Here's how the part is built. I have some questions about the finished solid (model axes, mm). Coordinates: 2 decimals unless noted, no trailing zeros. Write each loop counter-clockwise with the first axis right and the second up, starting at its lowest first coordinate (ties: lowest second). Pieces come first, ordered by that corner, then holes.
```python
from build123d import *

# Parameters (mm, degrees)
SKETCH1_R           = 2.25
BOSS_EXTRUDE1_DEPTH = 3.18


with BuildPart() as part:
    # Sketch1 → Boss-Extrude1 (new body)
    with BuildSketch(Plane.XY):
        with BuildLine():
            ThreePointArc((22.5, 0), (15.998046756, 15.821267332), (0.25, 22.498611068))
            Line((0.25, 22.498611068), (0.25, -22.498611068))
            ThreePointArc((0.25, -22.498611068), (15.998046756, -15.821267332), (22.5, 0))
        make_face()
        with Locations(Location((9.25, -16.02146997, 0), (0, 0, 180))):
            Circle(SKETCH1_R, mode=Mode.SUBTRACT)
        with Locations(Location((18.5, 0, 0), (0, 0, 180))):
            Circle(SKETCH1_R, mode=Mode.SUBTRACT)
        with Locations(Location((9.25, 16.02146997, 0), (0, 0, 180))):
            Circle(SKETCH1_R, mode=Mode.SUBTRACT)
    extrude(amount=BOSS_EXTRUDE1_DEPTH)


solid = part.part
```
1) Will this pin go through, and if not, where does the flat tip stop? pin 1 (3.5 mm diameter, centred on x = 9.25, y = -16.02, fed in from -Z).
Values follow:
pin 1: passes through
2) We'd pull the mould along X, two halves only. Please class faces 1 (the face through (11.036, 17.391, 1.568)), 2 (the face through (9.738, -13.825, 1.568)), 3 (the face through (9, 0, 0)), 4 (the face through (0.25, 0, 2)): pulls with the +X half, pulls with the -X half, needs draft (parallel to the pull), parting line crosses it, or undercut.
Values follow:
face 1: undercut
face 2: undercut
face 3: needs draft
face 4: pulls with the -X half
3) Imagine slicing it at A-A on x = 9.25. Please give me the cut outline in (y, z), then the cut area to 3 significant figures.
Values follow:
outline: (-20.51, 0) - (-18.27, 0) - (-18.27, 3.18) - (-20.51, 3.18) - close; (-13.77, 0) - (13.77, 0) - (13.77, 3.18) - (-13.77, 3.18) - close; (18.27, 0) - (20.51, 0) - (20.51, 3.18) - (18.27, 3.18) - close
area: 102 mm2
4) I need wall thicknesses on probe 1 along Y at (x, z) = (9, 0.9); probe 2 along Y at (x, z) = (9.25, 0.7); probe 3 along X at (y, z) = (2, 0.3). Which ranges of each line are inside material? Lowest first, please.
Values follow:
probe 1: y = -20.62 to -18.26, -13.79 to 13.79, 18.26 to 20.62
probe 2: y = -20.51 to -18.27, -13.77 to 13.77, 18.27 to 20.51
probe 3: x = 0.25 to 17.47, 19.53 to 22.41
5) Imagine slicing it at B-B on x = 18.5. Please give me the cut outline in (y, z).
Values follow:
outline: (-12.81, 0) - (-2.25, 0) - (-2.25, 3.18) - (-12.81, 3.18) - close; (2.25, 0) - (12.81, 0) - (12.81, 3.18) - (2.25, 3.18) - close
6) Imagine slicing it at D-D on y = 19.5. Please give me the cut outline in (x, z).
Values follow:
outline: (0.25, 0) - (11.22, 0) - (11.22, 3.18) - (0.25, 3.18) - close
